Drawing for the job (mm, zero at the part's lowest x, y, z). A direction names the side the tool comes from. Coordinates: 2 decimals unless noted, no trailing zeros. Write each loop counter-clockwise with the first axis right and the second up, starting at its lowest first coordinate (ties: lowest second). Pieces come first, ordered by that corner, then holes. Notation, with made-up numbers: M -39,68 L 1,68 A16 ccw 1,76 Z; hole C -33.75,63.25 d3. An arc over 180 degrees is marked long. Put each result on its own line as item: value. Start each with the question number.
Q1. Cut at D-D (z = 65.5). Write the cut outline in (x, y).
Q2. Pull direction X, two halves, no side cores. Call the marked faces 4, 5 and 6: pulls with the +X half, pulls with the -X half, needs draft (parallel to the pull), parting line crosses it, or undercut.
Q3. Drill centre lines: line 1 along Z through (x, y) = (15, 4); line 2 along Y through (x, z) = (88, 66.25); line 3 along Z through (x, y) = (94, 3). Where is each one in solid material? Low to high.
Q4. Cut at C-C (x = 86.5). Write the cut outline in (y, z), then the cut area to 3 significant figures.
Q5. Which spindle directions (+Z, -Z, +X, -X, +Y, -Y) get a long thin tool onto all of the face, cutting with end or side? Do the marked faces 1, 2 and 3. Say none if no direction does.
Q6. Drop flat-ended pins along their axis: pin 1 (2 mm diameter, centred on x = 45.5, z = 90.5, fed in from -Y); pin 2 (5 mm diameter, centred on x = 88, z = 38.5, fed in from +Y); pin 3 (6 mm diameter, centred on x = 23, y = 24, fed in from -Z). Give the stop position or say it passes through.
Q7. Cut at A-A (y = 29.5). Write the cut outline in (x, z).
Q8. Cut at B-B (z = 45). Write the cut outline in (x, y).
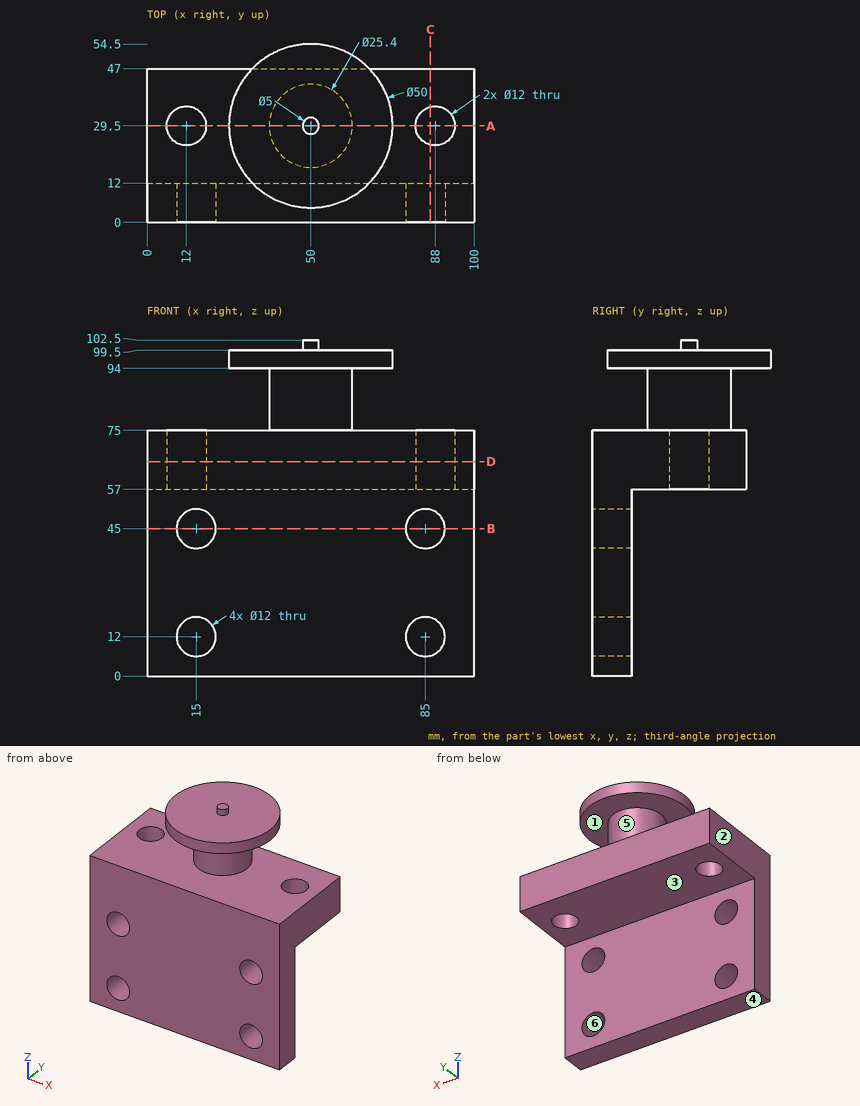
Computed values:
1. outline: M 0,0 L 100,0 L 100,47 L 0,47 Z; hole C 12,29.5 d12; hole C 88,29.5 d12
2. face 4: needs draft
2. face 5: parting line crosses it
2. face 6: undercut
3. line 1: 0 to 6, 18 to 39, 51 to 75
3. line 2: 0 to 23.5, 35.5 to 47
3. line 3: 0 to 75
4. outline: M 0,0 L 12,0 L 12,6.19 L 0,6.19 Z; M 0,17.81 L 12,17.81 L 12,39.19 L 0,39.19 Z; M 0,50.81 L 12,50.81 L 12,57 L 23.69,57 L 23.69,75 L 0,75 Z; M 35.31,57 L 47,57 L 47,75 L 35.31,75 Z
4. area: 1,040 mm2
5. face 1: none
5. face 2: +Z, -Z, -X, +Y, -Y
5. face 3: -Z, +X, -X, +Y
6. pin 1: y = 17.29
6. pin 2: y = 12
6. pin 3: z = 57
7. outline: M 0,57 L 6,57 L 6,75 L 0,75 Z; M 18,57 L 82,57 L 82,75 L 62.7,75 L 62.7,94 L 75,94 L 75,99.5 L 52.5,99.5 L 52.5,102.5 L 47.5,102.5 L 47.5,99.5 L 25,99.5 L 25,94 L 37.3,94 L 37.3,75 L 18,75 Z; M 94,57 L 100,57 L 100,75 L 94,75 Z
8. outline: M 0,0 L 9,0 L 9,12 L 0,12 Z; M 21,0 L 79,0 L 79,12 L 21,12 Z; M 91,0 L 100,0 L 100,12 L 91,12 Z
